For this review, take the finished solid that the model builds, in its own axes (mm). A direction names the side the tool comes from. Round coordinates to 2 decimals unless told otherwise and drop trailing zeros. Order: outer loops, then holes, each group sorted by start corner. A loop starts at its lowest first (then second) coordinate and runs counter-clockwise, first axis right, second up. Notation, with made-up numbers: (-16, -21.5) - (-11, -21.5) arc R23 cw to (-11, 8.5) - close; hole circle Ø1 at (22.25, -1.75). An arc over 180 degrees is marked (long way). Write each question's results on one line, items separated by ' | '. Start each with the question number.
(1) Draft analysis for pull direction Y (two halves, no side actions). For faces 6 (the cylindrical face through (3.09, -2.67, -7.08)), 7 (the flat face through (-5, 0, -16)), 8 (the cylindrical face through (-0.596, -4.312, -0.38)), 9 (the cylindrical face through (-0.49, -0.63, -25.02)), state which applies: pulls with the +Y half, pulls with the -Y half, needs draft (parallel to the pull), parting line crosses it, or undercut.
(2) For L1, parallel to Z at x = 3.75, y = 3.25; L2, parallel to Z at x = 1, y = -0.75; L3, parallel to X at y = 0, z = -24.75, list the stretches that pass through material, from the lowest coordinate up. Write a range as from..to.
(3) Take a section at C-C, the plane x = -3.5. Give the boundary of the cut face in (y, z).
(4) For faces 1 (the cylindrical face through (-2.44, -0.54, -24.74)), 2 (the flat face through (-4, 5, -9)), 3 (the cylindrical face through (0, 6, -16)), 4 (the flat face through (-4, -5, -9)), 5 (the flat face through (0, 0, -0.8)), list the 3-axis set-ups (+Z, -Z, +X, -X, +Y, -Y) from which the entire face can be reached by the end or side of a thin tool; tool diameter is ignored.
(5) Take a section at B-B, the plane z = -4. Give the boundary of the cut face in (x, y).
(6) Take a section at A-A, the plane y = 0. Give the number of separate pieces and of enclosed holes in the cut face, plus the area to 3 significant figures.
(7) Insertion check: pin 1 Ø4 at (y, z) = (3.5, 5) entering from -X; pin 2 Ø1.3 at (x, y) = (-1.5, -5) entering from -Z; pin 3 Ø1.1 at (x, z) = (-0.5, 3.5) entering from +Y; pin 4 Ø1 at (x, y) = (0, -4.5) entering from +Z. Each pin has a flat end and moves straight along its axis. Give the tip position at first contact, or say it passes through.
```python
from build123d import *

# Parameters (mm, degrees)
SKETCH1_W                    = 10
SKETCH1_H                    = 12
BOSS_EXTRUDE1_DEPTH          = 9
BOSS_EXTRUDE2_DEPTH          = 15
CUT_EXTRUDE1_DEPTH           = 9
FILLET1_R                    = 0.75
M1_6X0_35_TAPPED_HOLE1_D     = 1.25
M1_6X0_35_TAPPED_HOLE1_DEPTH = 0.75
M1_6X0_35_TAPPED_HOLE1_TIP   = 0.375537887
CUT_EXTRUDE2_START           = -0.8
SKETCH7_W                    = 10
SKETCH7_H                    = 12
SKETCH7_R                    = 1.5
CUT_EXTRUDE2_DEPTH           = 4.25
CUT_EXTRUDE3_START           = -0.8
SKETCH8_W                    = 10
SKETCH8_H                    = 12
SKETCH8_R                    = 1.5
CUT_EXTRUDE3_DEPTH           = 2.5


with BuildPart() as part:
    # Sketch1 → Boss-Extrude1 (new body)
    with BuildSketch(Plane.XY):
        Rectangle(SKETCH1_W, SKETCH1_H)
    extrude(amount=-BOSS_EXTRUDE1_DEPTH)

    # Sketch2 → Boss-Extrude2 (add)
    with BuildSketch(Plane(origin=(0, 0, -9), x_dir=(-1, 0, 0), z_dir=(0, 0, -1))):
        with BuildLine():
            Line((-5, 3.31662479), (-5, -3.31662479))
            ThreePointArc((-5, -3.31662479), (0, -6), (5, -3.31662479))
            Line((5, -3.31662479), (5, 3.31662479))
            ThreePointArc((5, 3.31662479), (0, 6), (-5, 3.31662479))
        make_face()
    extrude(amount=BOSS_EXTRUDE2_DEPTH)

    # Sketch3 → Revolve1 (revolve)
    with BuildSketch(Plane(origin=(0, 0, 0), x_dir=(0, 0, -1), z_dir=(1, 0, 0))):
        Polygon((-10, 0), (30, 0), (30, 0.5), (24.524329041, 0.5), (24.524329041, 0.797163214), (25.5, 0.797163214), (25.5, 2.5), (0, 2.5), (0, 1.95), (-0.6, 1.95), (-0.6, 1.5), (-10, 1.5), align=None)
    revolve(axis=Axis((0, 0, 10), (0, 0, -1)))

    # Sketch4 → Cut-Extrude1 (cut)
    with BuildSketch(Plane.XY.offset(10)):
        with BuildLine():
            Line((1.118033989, 1), (-1.118033989, 1))
            ThreePointArc((-1.118033989, 1), (0, 1.5), (1.118033989, 1))
        make_face()
    extrude(amount=-CUT_EXTRUDE1_DEPTH, mode=Mode.SUBTRACT)

    # Fillet1
    fillet1_edges = [part.edges().sort_by_distance(p)[0] for p in [
        (-5, -6, -4.5),
        (5, -6, -4.5),
        (5, 6, -4.5),
        (-5, 6, -4.5),
    ]]
    fillet(fillet1_edges, radius=FILLET1_R)

    # M1.6x0.35 Tapped Hole1
    with Locations(Plane.XY):
        with Locations((0, -4.5), (0, 4.5)):
            Hole(M1_6X0_35_TAPPED_HOLE1_D / 2, depth=M1_6X0_35_TAPPED_HOLE1_DEPTH)
            with Locations((0, 0, -(M1_6X0_35_TAPPED_HOLE1_DEPTH + M1_6X0_35_TAPPED_HOLE1_TIP / 2))):  # 118° drill point
                Cone(0, M1_6X0_35_TAPPED_HOLE1_D / 2, M1_6X0_35_TAPPED_HOLE1_TIP, mode=Mode.SUBTRACT)

    # Sketch7 → Cut-Extrude2 (cut)
    with BuildSketch(Plane.XY.offset(CUT_EXTRUDE2_START)):
        Rectangle(SKETCH7_W, SKETCH7_H)
        with Locations((-3.151875275, 4.232117394)):
            Circle(SKETCH7_R, mode=Mode.SUBTRACT)
        with Locations((3.282813714, -4.157295429)):
            Circle(SKETCH7_R, mode=Mode.SUBTRACT)
    extrude(amount=-CUT_EXTRUDE2_DEPTH, mode=Mode.SUBTRACT)

    # Sketch8 → Cut-Extrude3 (cut)
    with BuildSketch(Plane.XY.offset(-5.05).offset(CUT_EXTRUDE3_START)):
        Rectangle(SKETCH8_W, SKETCH8_H)
        with Locations((-3.151875275, 4.232117394)):
            Circle(SKETCH8_R, mode=Mode.SUBTRACT)
        with Locations((3.282813714, -4.157295429)):
            Circle(SKETCH8_R, mode=Mode.SUBTRACT)
    extrude(amount=-CUT_EXTRUDE3_DEPTH, mode=Mode.SUBTRACT)


solid = part.part
```
Results below:
1) face 6: parting line crosses it | face 7: needs draft | face 8: undercut | face 9: undercut
2) L1: z = -24..-8.35, -5.85..-5.05, -0.8..0 | L2: z = -25.5..-8.35, -5.85..-5.05, -0.8..10 | L3: x = -2.5..-0.8, -0.5..0.5, 0.8..2.5
3) outline: (-6, -9) - (-4.87, -9) - (-4.87, -24) - (4.87, -24) - (4.87, -9) - (6, -9) - (6, -8.35) - (5.69, -8.35) - (5.69, -5.85) - (6, -5.85) - (6, -5.05) - (5.69, -5.05) - (5.69, -0.8) - (6, -0.8) - (6, 0) - (-6, 0) - (-6, -0.8) - (2.77, -0.8) - (2.77, -5.05) - (-6, -5.05) - (-6, -5.85) - (2.77, -5.85) - (2.77, -8.35) - (-6, -8.35) - close
4) face 1: -Z | face 2: -Z, -X, +Y | face 3: -Z, +Y | face 4: -Z, -X, -Y | face 5: none
5) outline: circle Ø3 at (-3.15, 4.23); circle Ø3 at (3.28, -4.16)
6) separate pieces: 3 | enclosed holes: 0 | area: 214 mm^2
7) pin 1: passes through | pin 2: stops at z = -24 | pin 3: stops at y = 1 | pin 4: stops at z = -5.05
